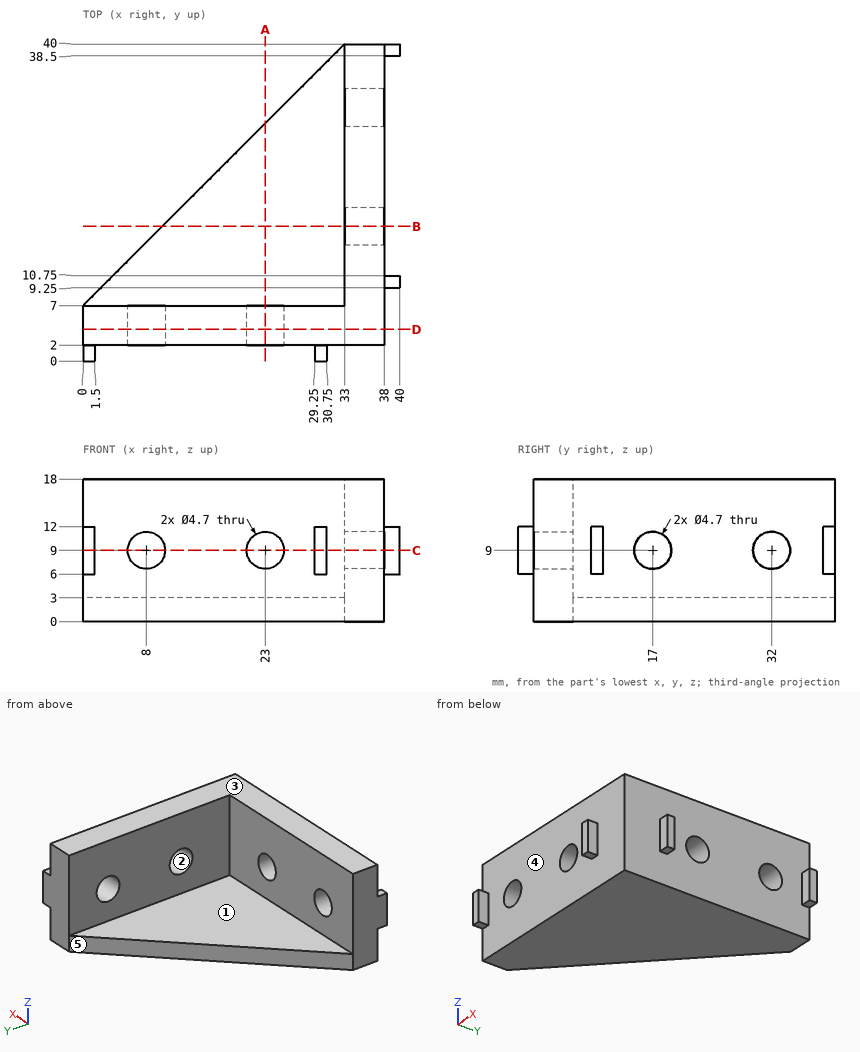
Part print with two shaded views. Sizes in mm from the minimum x, y, z corner. A direction names the side the tool comes from. Coordinates: 2 decimals unless noted, no trailing zeros. Write each loop counter-clockwise with the first axis right and the second up, starting at its lowest first coordinate (ties: lowest second). Pieces come first, ordered by that corner, then holes.
(1) Cut at C-C on z = 9. State how many separate pieces and enclosed holes the cut face has, and give its area (3 significant figures).
(2) Mould opens along X. For the marked faces 3, 4 and 5 say: pulls with the +X half, pulls with the -X half, needs draft (parallel to the pull), parting line crosses it, or undercut.
(3) Cut at A-A on x = 23. List the corners of the cut face in (y, z), and give its area (4 significant figures).
(4) 3-axis set-ups, long thin cutter, end or side, ignore diameter. For the marked faces 1 and 2: which of +Z, -Z, +X, -X, +Y, -Y reach the whole face in a straight line?
(5) Drill centre lines: line 1 (X direction, y = 3.65, z = 9); line 2 (Y direction, x = 35.8, z = 9); line 3 (Z direction, x = 35, y = 32). Where is each one in solid material? Low to high.
(6) Cut at D-D on y = 4. List the corners of the cut face in (x, z), and give its area (3 significant figures).
(7) Cut at B-B on y = 17. List the corners of the cut face in (x, z), and give its area (4 significant figures).
(8) Pin check, flat tips, straight feed: pin 1 Ø7.5 at (y, z) = (25, 13) entering from -X; pin 2 Ø5.5 at (x, z) = (26, 12.5) entering from -Y; pin 3 Ø10 at (x, z) = (10, 7) entering from +Y; pin 4 Ø3 at (x, z) = (8, 9) entering from +Y. Stop position of each tip, or through.
Working result:
1. separate pieces: 5
1. enclosed holes: 0
1. area: 273 mm2
2. face 3: needs draft
2. face 4: undercut
2. face 5: pulls with the -X half
3. outline: (2, 0) - (30, 0) - (30, 3) - (7, 3) - (7, 6.65) - (2, 6.65) - close; (2, 11.35) - (7, 11.35) - (7, 18) - (2, 18) - close
3. area: 135.5 mm2
4. face 1: +Z, -X, +Y
4. face 2: +X, -X
5. line 1: x = 0 to 5.65, 10.35 to 20.65, 25.35 to 38
5. line 2: y = 2 to 14.65, 19.35 to 29.65, 34.35 to 40
5. line 3: z = 0 to 6.65, 11.35 to 18
6. outline: (0, 0) - (38, 0) - (38, 18) - (0, 18) - close; hole circle Ø4.7 at (8, 9); hole circle Ø4.7 at (23, 9)
6. area: 649 mm2
7. outline: (10, 0) - (38, 0) - (38, 6.65) - (33, 6.65) - (33, 3) - (10, 3) - close; (33, 11.35) - (38, 11.35) - (38, 18) - (33, 18) - close
7. area: 135.5 mm2
8. pin 1: stops at x = 33
8. pin 2: stops at y = 2
8. pin 3: stops at y = 20
8. pin 4: passes through
